from build123d import *

# Parameters (mm, degrees)
BOSS_EXTRUDE1_DEPTH = 0.1
SKETCH2_R           = 0.2
BOSS_EXTRUDE2_DEPTH = 1
SKETCH3_R           = 3
BOSS_EXTRUDE3_DEPTH = 0.3
SKETCH4_R           = 0.15
CUT_EXTRUDE1_DEPTH  = 2.4


with BuildPart() as part:
    # Sketch1 → Boss-Extrude1 (new body)
    with BuildSketch(Plane(origin=(0, 0, 0), x_dir=(1, 0, 0), z_dir=(0, 1, 0))):
        with BuildLine():
            Line((-0.127585763, 0.586277983), (-0.127585763, 1.500996355))
            add(Edge.make_bspline(
                [(-0.127585763, 1.500996355), (-0.613609966, 1.292745221), (-0.997428455, 1.836597424), (-0.58121193, 3.118510404), (-0.267201121, 3.648320045)],
                knots=[0, 0, 0, 0, 0.463523694, 0.927047389, 0.927047389, 0.927047389, 0.927047389], degree=3))
            ThreePointArc((-0.267201121, 3.648320045), (-0.239390751, 3.74285385), (-0.260097073, 3.83919338))
            Line((-0.260097073, 3.83919338), (-0.359543258, 4.039599684))
            ThreePointArc((-0.359543258, 4.039599684), (-0.36190456, 4.065500923), (-0.338780115, 4.077405124))
            Line((-0.338780115, 4.077405124), (-0.157398308, 4.077405124))
            ThreePointArc((-0.157398308, 4.077405124), (-0.122926977, 4.092023881), (-0.108734749, 4.126672999))
            Line((-0.108734749, 4.126672999), (-0.080541531, 8.433581196))
            Line((-0.080541531, 8.433581196), (0.080699272, 8.433581196))
            Line((0.080699272, 8.433581196), (0.109905863, 4.115918774))
            ThreePointArc((0.109905863, 4.115918774), (0.126940207, 4.088385312), (0.157398308, 4.077405124))
            Line((0.157398308, 4.077405124), (0.338780115, 4.077405124))
            ThreePointArc((0.338780115, 4.077405124), (0.36190456, 4.065500923), (0.359543258, 4.039599684))
            Line((0.359543258, 4.039599684), (0.260097073, 3.83919338))
            ThreePointArc((0.260097073, 3.83919338), (0.239390751, 3.74285385), (0.267201121, 3.648320045))
            add(Edge.make_bspline(
                [(0.127585763, 1.500996355), (1.09963417, 1.084494086), (0.895222739, 2.588700762), (0.267201121, 3.648320045)],
                knots=[0, 0, 0, 0, 0.927047389, 0.927047389, 0.927047389, 0.927047389], degree=3))
            Line((0.127585763, 1.500996355), (0.127585763, 0.586277983))
            ThreePointArc((0.127585763, 0.586277983), (0, -0.6), (-0.127585763, 0.586277983))
        make_face()
        with BuildLine():
            Line((0.113918239, 3.522473584), (0.125824318, 1.761520463))
            add(Edge.make_bspline(
                [(0.125824318, 1.761520463), (0.890796605, 1.231501017), (0.501435582, 2.785705467), (0.113918239, 3.522473584)],
                knots=[0.044229807, 0.044229807, 0.044229807, 0.044229807, 0.913901264, 0.913901264, 0.913901264, 0.913901264], degree=3))
        make_face(mode=Mode.SUBTRACT)
        with BuildLine():
            Line((-0.113060898, 3.524102277), (-0.125714788, 1.761596361))
            add(Edge.make_bspline(
                [(-0.125714788, 1.761596361), (-0.891397992, 1.23096165), (-0.500879166, 2.787963848), (-0.113060898, 3.524102277)],
                knots=[0.044188303, 0.044188303, 0.044188303, 0.044188303, 0.914542619, 0.914542619, 0.914542619, 0.914542619], degree=3))
        make_face(mode=Mode.SUBTRACT)
    extrude(amount=BOSS_EXTRUDE1_DEPTH)

    # Sketch2 → Boss-Extrude2 (add)
    with BuildSketch(Plane.XZ):
        Circle(SKETCH2_R)
    extrude(amount=BOSS_EXTRUDE2_DEPTH)

    # Sketch3 → Boss-Extrude3 (add)
    with BuildSketch(Plane.XZ.offset(1)):
        Circle(SKETCH3_R)
    extrude(amount=BOSS_EXTRUDE3_DEPTH)

    # Sketch4 → Cut-Extrude1 (cut, through all)
    with BuildSketch(Plane(origin=(0, 0.1, 0), x_dir=(1, 0, 0), z_dir=(0, 1, 0))):
        Circle(SKETCH4_R)
    extrude(amount=-CUT_EXTRUDE1_DEPTH, mode=Mode.SUBTRACT)


solid = part.part
The listing builds one solid part. Answer for the finished solid, in the listing's coordinates (mm). Coordinates: 2 decimals unless noted, no trailing zeros. Order: outer loops, then holes, each group sorted by start corner. A loop starts at its lowest first (then second) coordinate and runs counter-clockwise, first axis right, second up. Notation, with made-up numbers: (-4.5, 68) -> (7.5, 68) arc R5 cw to (7.5, 75) -> close; hole circle Ø8 at (16.5, 80.5). An arc over 180 degrees is marked (long way). Answer in a Markdown table with one row per item. Add a question column.
Item 1: Find section B-B (y = -0.4). Write down the section's boundary in (x, z), then the cut area to 3 significant figures.
Item 2: Find section A-A (z = 0). Write down the section's boundary in (x, y), then the cut area to 3 significant figures.
Item 3: Find section C-C (x = 1.8). Write down the section's boundary in (y, z).
Item 4: Find the intervals of material crossed by L1, parallel to Y at x = 0.8, z = 1.25; L2, parallel to X at y = -1.05, z = -2.75; L3, parallel to Z at x = -2.4, y = -1.2, in increasing order. Write a range as from..to.
Item 5: Find section D-D (z = 2). Write down the section's boundary in (x, y).
Item 6: Each of these flat-tipped pins is pushed along its axis until it touches: P1, Ø2, axis at x = 2, z = 1, coming from the +Y side; P2, Ø1.8, axis at x = 0, z = -4, coming from the -Y side; P3, Ø1.8, axis at x = 1, z = -1.5, coming from the +Y side. Where does it stop, or does it pass through?
Result set:
| question | item | result |
|---|---|---|
| 1 | outline | circle Ø0.4 at (0, 0); hole circle Ø0.3 at (0, 0) |
| 1 | area | 0.0550 mm² |
| 2 | outline | (-3, -1.3) -> (-0.15, -1.3) -> (-0.15, 0.1) -> (-0.6, 0.1) -> (-0.6, 0) -> (-0.2, 0) -> (-0.2, -1) -> (-3, -1) -> close; (0.15, -1.3) -> (3, -1.3) -> (3, -1) -> (0.2, -1) -> (0.2, 0) -> (0.6, 0) -> (0.6, 0.1) -> (0.15, 0.1) -> close |
| 2 | area | 1.90 mm² |
| 3 | outline | (-1.3, -2.4) -> (-1, -2.4) -> (-1, 2.4) -> (-1.3, 2.4) -> close |
| 4 | L1 | y = -1.3..-1 |
| 4 | L2 | x = -1.2..1.2 |
| 4 | L3 | z = -1.8..1.8 |
| 5 | outline | (-2.24, -1.3) -> (2.24, -1.3) -> (2.24, -1) -> (-2.24, -1) -> close |
| 6 | P1 | stops at y = -1 |
| 6 | P2 | stops at y = 0 |
| 6 | P3 | stops at y = 0.1 |
